Model file for the job. Use its own axes, mm. A direction names the side the tool comes from. Round coordinates to 2 decimals unless told otherwise and drop trailing zeros. Loops run counter-clockwise (first coordinate to the right, second up) from the corner with the lowest first, then second, coordinate; pieces in that order, holes last.
from build123d import *

# Parameters (mm, degrees)
SKETCH_1_R          = 5
EXTRUDE_1_DEPTH     = 10
SKETCH_2_W          = 20
SKETCH_2_H          = 10
EXTRUDE_2_DEPTH     = 50
CUT_EXTRUDE_1_DEPTH = 50
SKETCH_5_W          = 10
SKETCH_5_H          = 30
EXTRUDE_3_DEPTH     = 50
SKETCH_6_W          = 10
SKETCH_6_H          = 30
EXTRUDE_4_DEPTH     = 55
SKETCH_7_R          = 15
SKETCH_7_R_2        = 10
EXTRUDE_5_DEPTH     = 20
SKETCH_8_R          = 15
EXTRUDE_6_DEPTH     = 10


with BuildPart() as part:
    # 草圖1 → 填料-伸長1 (new body)
    with BuildSketch(Plane.XY):
        with BuildLine():
            Line((15, 20), (15, -20))
            ThreePointArc((15, -20), (0, -35), (-15, -20))
            Line((-15, -20), (-15, 20))
            ThreePointArc((-15, 20), (0, 35), (15, 20))
        make_face()
        with Locations((0, -20)):
            Circle(SKETCH_1_R, mode=Mode.SUBTRACT)
        with Locations((0, 20)):
            Circle(SKETCH_1_R, mode=Mode.SUBTRACT)
    extrude(amount=EXTRUDE_1_DEPTH)

    # 草圖2 → 填料-伸長2 (add)
    with BuildSketch(Plane.XY.offset(10)):
        with Locations((5, 0)):
            Rectangle(SKETCH_2_W, SKETCH_2_H)
    extrude(amount=EXTRUDE_2_DEPTH)

    # 草圖4 → 除料-伸長1 (cut)
    with BuildSketch(Plane.XZ.offset(5)):
        Polygon((-5, 60), (15, 10), (15, 60), align=None)
    extrude(amount=-CUT_EXTRUDE_1_DEPTH, mode=Mode.SUBTRACT)

    # 草圖5 → 填料-伸長3 (add)
    with BuildSketch(Plane.XY.offset(10)):
        with Locations((-10, 0)):
            Rectangle(SKETCH_5_W, SKETCH_5_H)
    extrude(amount=EXTRUDE_3_DEPTH)

    # 草圖6 → 填料-伸長4 (add)
    with BuildSketch(Plane.ZY.offset(15)):
        with Locations((55, 0)):
            Rectangle(SKETCH_6_W, SKETCH_6_H)
    extrude(amount=EXTRUDE_4_DEPTH)

    # 草圖7 → 填料-伸長5 (add)
    with BuildSketch(Plane.XY.offset(60)):
        with Locations(Location((-70, 0, 0), (0, 0, 270))):
            Circle(SKETCH_7_R)
        with Locations(Location((-70, 0, 0), (0, 0, 90))):
            Circle(SKETCH_7_R_2, mode=Mode.SUBTRACT)
    extrude(amount=EXTRUDE_5_DEPTH)

    # 草圖8 → 填料-伸長6 (add)
    with BuildSketch(Plane(origin=(0, 0, 50), x_dir=(-1, 0, 0), z_dir=(0, 0, -1))):
        with Locations(Location((70, 0, 0), (0, 0, 90))):
            Circle(SKETCH_8_R)
    extrude(amount=-EXTRUDE_6_DEPTH)


solid = part.part
Q1. Slice it at B-B on z = 26.5. Give the cut face in (x, y), plus the area to 3 significant figures.
Q2. Slice it at D-D on x = -76. Give the cut face in (y, z).
Q3. Tool access for faces 4 (the face through (-50, 0, 50)), 5 (the face through (-23, -15, 52)), 6 (the face through (-5, -10, 35)), 7 (the face through (-5, 10, 35)): list every direction of +Z, -Z, +X, -X, +Y, -Y with a clear straight run to the whole face (end or side of a thin tool).
Q4. Probe line 1 (Y direction, x = 0, z = 3); line 2 (X direction, y = 0, z = 67); line 3 (X direction, y = -9, z = 28). List the from-to ranges inside material, lowest first.
Q5. Pull direction X, two halves, no side cores. Call faces 1 (the face through (-1.08, -24.88, 4.93)), 2 (the face through (-23, 15, 52)), 3 (the face through (15, 0, 5)): pulls with the +X half, pulls with the -X half, needs draft (parallel to the pull), parting line crosses it, or undercut.
Q6. Flat gauge pins, fed straight in: P1, Ø9, axis at x = 1.5, y = -18.5, coming from the +Z side; P2, Ø1.5, axis at x = -46, z = 56.5, coming from the -Y side; P3, Ø4, axis at y = -14.5, z = 33.5, coming from the +X side; P4, Ø11, axis at x = -62.5, y = 4.5, coming from the +Z side. Where does each tip first touch, or does it go through?
Q7. Slice it at A-A on x = 0. Give the cut face in (y, z), plus the area to 3 significant figures.
Q8. Slice it at C-C on y = 17.5. Give the cut face in (x, z).
Reply:
1. outline: (-15, -15) - (-5, -15) - (-5, -5) - (8.4, -5) - (8.4, 5) - (-5, 5) - (-5, 15) - (-15, 15) - close
1. area: 434 mm2
2. outline: (-13.75, 50) - (13.75, 50) - (13.75, 80) - (8, 80) - (8, 60) - (-8, 60) - (-8, 80) - (-13.75, 80) - close
3. face 4: -Z, -X, +Y, -Y
3. face 5: +Z, +X, -X, -Y
3. face 6: +Z, +X, -Y
3. face 7: +Z, +X, +Y
4. line 1: y = -35 to -25, -15 to 15, 25 to 35
4. line 2: x = -85 to -80, -60 to -55
4. line 3: x = -15 to -5
5. face 1: undercut
5. face 2: needs draft
5. face 3: pulls with the +X half
6. P1: stops at z = 10
6. P2: stops at y = -15
6. P3: stops at x = -5
6. P4: stops at z = 80
7. outline: (-35, 0) - (-25, 0) - (-25, 10) - (-35, 10) - close; (-15, 0) - (15, 0) - (15, 10) - (5, 10) - (5, 47.5) - (-5, 47.5) - (-5, 10) - (-15, 10) - close; (25, 0) - (35, 0) - (35, 10) - (25, 10) - close
7. area: 875 mm2
8. outline: (-15, 0) - (-4.33, 0) - (-4.33, 10) - (-15, 10) - close; (4.33, 0) - (15, 0) - (15, 10) - (4.33, 10) - close
